from build123d import *

# Parameters (mm, degrees)
F0_R      = 60
F1_DEPTH  = 160
F2_R      = 115
F3_DEPTH  = 50
F4_R      = 160
F5_DEPTH  = 18
F6_SIZE   = 5
F7_R      = 42.875
F8_DEPTH  = 86
F9_R      = 27
F10_DEPTH = 430


with BuildPart() as f1:
    # F0 (on Front) → F1 (new body)
    with BuildSketch(Plane.XZ):
        Circle(F0_R)
    extrude(amount=F1_DEPTH)

    # F2 (on face) → F3 (join)
    with BuildSketch(Plane.XZ.offset(160)):
        Circle(F2_R)
    extrude(amount=F3_DEPTH)

    # F4 (on face) → F5 (join)
    with BuildSketch(Plane.XZ.offset(210)):
        Circle(F4_R)
    extrude(amount=F5_DEPTH)

    # F6
    f6_edges = [f1.edges().sort_by_distance(p)[0] for p in [
        (-115, -160, 0),
    ]]
    chamfer(f6_edges, length=F6_SIZE)

    # F7 (on face) → F8 (join)
    with BuildSketch(Plane(origin=(0, 0, 0), x_dir=(-1, 0, 0), z_dir=(0, 1, 0))):
        Circle(F7_R)
    extrude(amount=F8_DEPTH)

    # F9 (on face) → F10 (cut)
    with BuildSketch(Plane(origin=(0, 86, 0), x_dir=(-1, 0, 0), z_dir=(0, 1, 0))):
        Circle(F9_R)
    extrude(amount=-F10_DEPTH, mode=Mode.SUBTRACT)


solid = f1.part
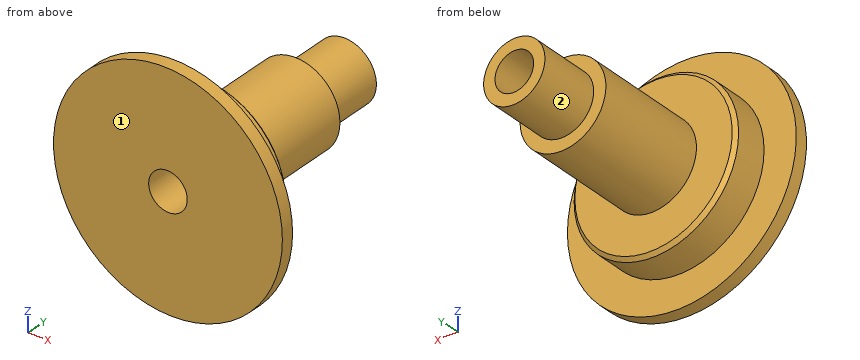
The listing builds one solid part. Answer for the finished solid, in the listing's coordinates (mm). Face numbers are marked on the shaded views. A direction names the side the tool comes from. Round coordinates to 2 decimals unless told otherwise and drop trailing zeros. Write each loop counter-clockwise with the first axis right and the second up, starting at its lowest first coordinate (ties: lowest second). Pieces come first, ordered by that corner, then holes. Notation, with made-up numbers: (75.5, 39) - (98.5, 39) arc R14 cw to (98.5, 64) - close; hole circle Ø4 at (-35.75, -30). An arc over 180 degrees is marked (long way). Use a Markdown table: item, result. Add a question column.
1. The part is cut by section A-A (x = 0). Write down the section's boundary in (y, z) (3 decimals).
2. A tool of negligible diameter and unlimited length cuts with its end or side. For the marked faces 1 and 2, from which of +Z, -Z, +X, -X, +Y, -Y can it reach the whole face along a straight path? Write none if from no direction.
3. The part is cut by section D-D (y = 40.5). Write down the section's boundary in (x, z) (3 decimals).
4. Consider line 1 (Z direction, x = 0, y = -57); line 2 (Z direction, x = 0, y = 16.5) (3 decimals); line 3 (Y direction, x = 11, z = 72). Determine where each line is inside the solid, lowest interval first.
5. The part is cut by section B-B (z = 0). Write down the section's boundary in (x, y) (3 decimals), and give its area (3 significant figures).
6. Flat-ended cylindrical pins translate along their axes: P1, Ø4, axis at y = -181.5, z = -15.5, coming from the +X side; P2, Ø8, axis at x = -34.5, y = -173, coming from the +Z side; P3, Ø8, axis at x = 19, y = -175.5, coming from the -Z side. Find the tip coordinate at first contact, or state that the pin passes through.
7. The part is cut by section C-C (y = -150.5). Write down the section's boundary in (x, z).
Reported:
| question | item | result |
|---|---|---|
| 1 | outline | (-228, -160) - (-210, -160) - (-210, -115) - (-165, -115) - (-160, -110) - (-160, -60) - (0, -60) - (0, -42.875) - (86, -42.875) - (86, -27) - (-228, -27) - close; (-228, 27) - (86, 27) - (86, 42.875) - (0, 42.875) - (0, 60) - (-160, 60) - (-160, 110) - (-165, 115) - (-210, 115) - (-210, 160) - (-228, 160) - close |
| 2 | face 1 | +Z, -Z, +X, -X, -Y |
| 2 | face 2 | +Y |
| 3 | outline | circle Ø85.75 at (0, 0); hole circle Ø54 at (0, 0) |
| 4 | line 1 | -60 to -27, 27 to 60 |
| 4 | line 2 | -42.875 to -27, 27 to 42.875 |
| 4 | line 3 | -228 to -160 |
| 5 | outline | (-160, -228) - (-27, -228) - (-27, 86) - (-42.875, 86) - (-42.875, 0) - (-60, 0) - (-60, -160) - (-110, -160) - (-115, -165) - (-115, -210) - (-160, -210) - close; (27, -228) - (160, -228) - (160, -210) - (115, -210) - (115, -165) - (110, -160) - (60, -160) - (60, 0) - (42.875, 0) - (42.875, 86) - (27, 86) - close |
| 5 | area | 26,900 mm^2 |
| 6 | P1 | x = 114.2 |
| 6 | P2 | z = 110.88 |
| 6 | P3 | z = -114.02 |
| 7 | outline | circle Ø120 at (0, 0); hole circle Ø54 at (0, 0) |
